Answer from the drawing. Dimensions are ordinates in mm from the lowest x, y and z of the part. Coordinates: 2 decimals unless noted, no trailing zeros. Loops run counter-clockwise (first coordinate to the right, second up) from the corner with the lowest first, then second, coordinate; pieces in that order, holes last.
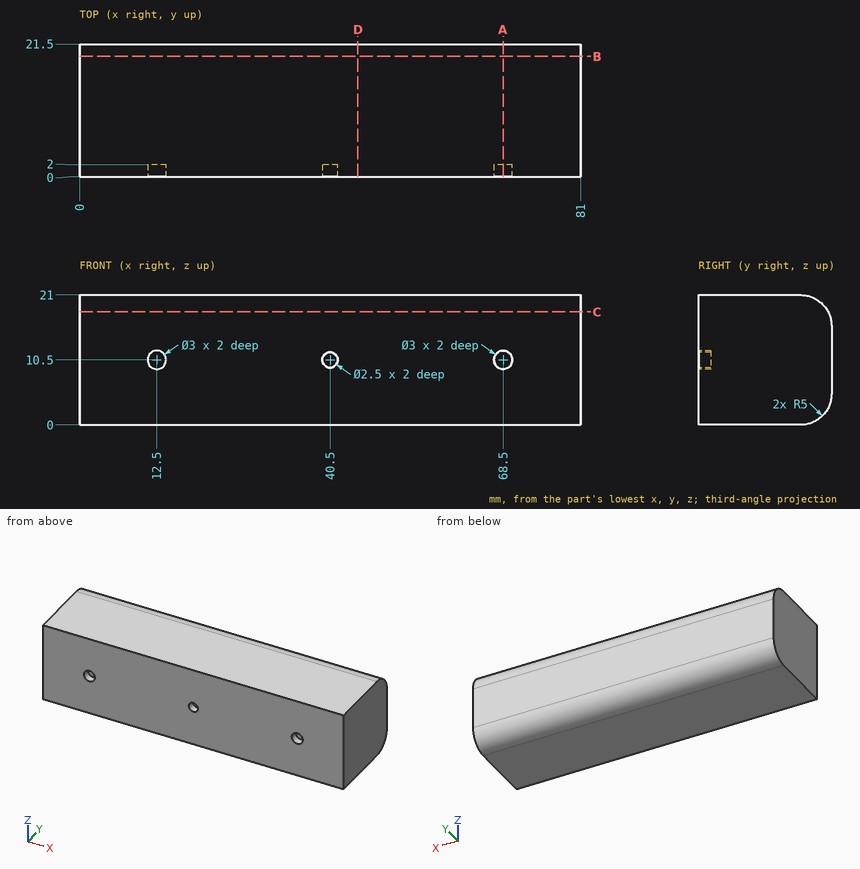
Item 1: A cutting plane is placed at A-A on x = 68.5. Determine the outline of the cut face in (y, z), then the cut area to 3 significant figures.
Numbers:
outline: (0, 0) - (16.5, 0) arc R5 ccw to (21.5, 5) - (21.5, 16) arc R5 ccw to (16.5, 21) - (0, 21) - (0, 12) - (2, 12) - (2, 9) - (0, 9) - close
area: 435 mm2
Item 2: A cutting plane is placed at B-B on y = 19.5. Determine the outline of the cut face in (x, z), then the cut area to 3 significant figures.
Numbers:
outline: (0, 1) - (81, 1) - (81, 20) - (0, 20) - close
area: 1,540 mm2
Item 3: A cutting plane is placed at D-D on x = 45. Determine the outline of the cut face in (y, z), then the cut area to 3 significant figures.
Numbers:
outline: (0, 0) - (16.5, 0) arc R5 ccw to (21.5, 5) - (21.5, 16) arc R5 ccw to (16.5, 21) - (0, 21) - close
area: 441 mm2
Item 4: Given pin 1 (2.5 mm diameter, centred on x = 12.5, z = 10.5, fed in from -Y); pin 2 (5 mm diameter, centred on x = 72, y = 17, fed in from -Z), each flat-ended and moving along its own axis, determine where each tip first touches the part or whether it passes through.
Numbers:
pin 1: stops at y = 2
pin 2: stops at z = 0
Item 5: A cutting plane is placed at C-C on z = 18.25. Determine the outline of the cut face in (x, y).
Numbers:
outline: (0, 0) - (81, 0) - (81, 20.97) - (0, 20.97) - close
Item 6: Find the intervals of material crossed by line 1 along Z through (x, y) = (12.5, 1.3); line 2 along Z through (x, y) = (40.5, 1); line 3 along Y through (x, z) = (57.5, 2.75), in increasing order.
Numbers:
line 1: z = 0 to 9, 12 to 21
line 2: z = 0 to 9.25, 11.75 to 21
line 3: y = 0 to 20.97
